The model under review builds one solid part; all positions refer to its coordinate system, in mm. A direction names the side the tool comes from. Give positions to 0.01 mm unless a question says otherwise; leave off trailing zeros. Order: outer loops, then holes, each group sorted by start corner. A loop starts at its lowest first (then second) coordinate and runs counter-clockwise, first axis right, second up.
```python
from build123d import *

# Parameters (mm, degrees)
F2_R            = 11.3641207455
F3_DEPTH        = 16
F5_DEPTH        = 16
F5_COPIES_COUNT = 15
F8_R            = 13.8641207455
F8_R_2          = 11.3641207455
F9_DEPTH        = 1.5
F7_R            = 4
F10_DEPTH       = 17.501
F11_R           = 13.8641207455
F11_R_2         = 11.4641207455
F12_DEPTH       = 0.1


# Not quite as in the source:
# - a feature of the source that left no trace in its solid (it failed there, or was rolled back) is left out
# - a pattern or mirror of a feature is missing from the dataset's text; its kind, count and spacing are read off the source's solid


with BuildPart() as f3:
    # F2 (on Top) → F3 (new body)
    with BuildSketch(Plane.XY):
        Circle(F2_R)
    extrude(amount=F3_DEPTH)

    # F4 (on face) → F5 (cut, through all)
    with BuildSketch(Plane.XY.offset(16)):
        with BuildLine():
            ThreePointArc((-2.0292576741, 11.181473678), (-1.6663457301, 11.0889370809), (-1.4991557657, 10.7538018594))
            ThreePointArc((-1.4991557657, 10.7538018594), (0, 9.3041207455), (1.4991557657, 10.7538018594))
            ThreePointArc((1.4991557657, 10.7538018594), (1.6663457301, 11.0889370809), (2.0292576741, 11.181473678))
            ThreePointArc((2.0292576741, 11.181473678), (0, 11.3641207455), (-2.0292576741, 11.181473678))
        make_face()
    f5 = extrude(amount=-F5_DEPTH, mode=Mode.SUBTRACT)

    # F5_copies: F5 ×15 about axis
    f5_copies_axis = Axis((0, 0, 0), (0, 0, 1))
    for i in range(1, F5_COPIES_COUNT):
        add(f5.rotate(f5_copies_axis, i * 360 / F5_COPIES_COUNT), mode=Mode.SUBTRACT)

    # F8 (on face) + F2 (on Top) → F9 (join)
    with BuildSketch(Plane.XY):
        Circle(F8_R)
        Circle(F8_R_2, mode=Mode.SUBTRACT)
    with BuildSketch(Plane.XY):
        Circle(F2_R)
    extrude(amount=-F9_DEPTH)

    # F7 (on face) → F10 (cut, through all)
    with BuildSketch(Plane.XY.offset(16)):
        Circle(F7_R)
    extrude(amount=-F10_DEPTH, mode=Mode.SUBTRACT)

    # F11 (on face) → F12 (join)
    with BuildSketch(Plane.XY):
        Circle(F11_R)
        Circle(F11_R_2, mode=Mode.SUBTRACT)
    extrude(amount=F12_DEPTH)


solid = f3.part
```
Item 1: Draft analysis for pull direction X (two halves, no side actions). For faces 1 (the cylindrical face through (6.893, 6.25, 8.112)), 2 (the flat face through (-8.3, 8.3, 0.1)), state which applies: released by +X, released by -X, zero draft, split by the parting line, or undercut.
Values found:
face 1: undercut
face 2: zero draft
Item 2: Take a section at A-A (y = 0). Give the boundary of the cut face in (x, z).
Values found:
outline: (-13.86, -1.5) - (-4, -1.5) - (-4, 16) - (-9.76, 16) - (-9.76, 0) - (-11.46, 0) - (-11.46, 0.1) - (-13.86, 0.1) - close; (4, -1.5) - (13.86, -1.5) - (13.86, 0.1) - (11.46, 0.1) - (11.46, 0) - (9.76, 0) - (9.76, 16) - (4, 16) - close
Item 3: For line 1 (Y direction, x = 0, z = 12.75); line 2 (X direction, y = 8.75, z = 14.5); line 3 (Z direction, x = -10.5, y = 9), list the stretches that pass through material, from the lowest coordinate up.
Values found:
line 1: y = -11.36 to -4, 4 to 9.3
line 2: x = -7.11 to -5.39, -3.4 to 3.4, 5.39 to 7.11
line 3: z = -1.5 to 0.1
Item 4: For faces 3 (the flat face through (3, -3, -1.5)), 4 (the cylindrical face through (-8.04, -4.68, 8.11)), list the 3-axis set-ups (+Z, -Z, +X, -X, +Y, -Y) from which the entire face can be reached by the end or side of a thin tool; tool diameter is ignored.
Values found:
face 3: -Z, +X, -X, +Y, -Y
face 4: +Z
Item 5: Clearance check with flat-ended pins moving along their axes: pin 1 Ø10 at (y, z) = (-5.5, 14) entering from -X; pin 2 Ø2 at (x, z) = (-5.5, 8.5) entering from +Y; pin 3 Ø10 at (x, z) = (6, 6) entering from -Y. State where each tip first meets the part, or that it passes through.
Values found:
pin 1: stops at x = -10.93
pin 2: stops at y = 9.47
pin 3: stops at y = -10.55
